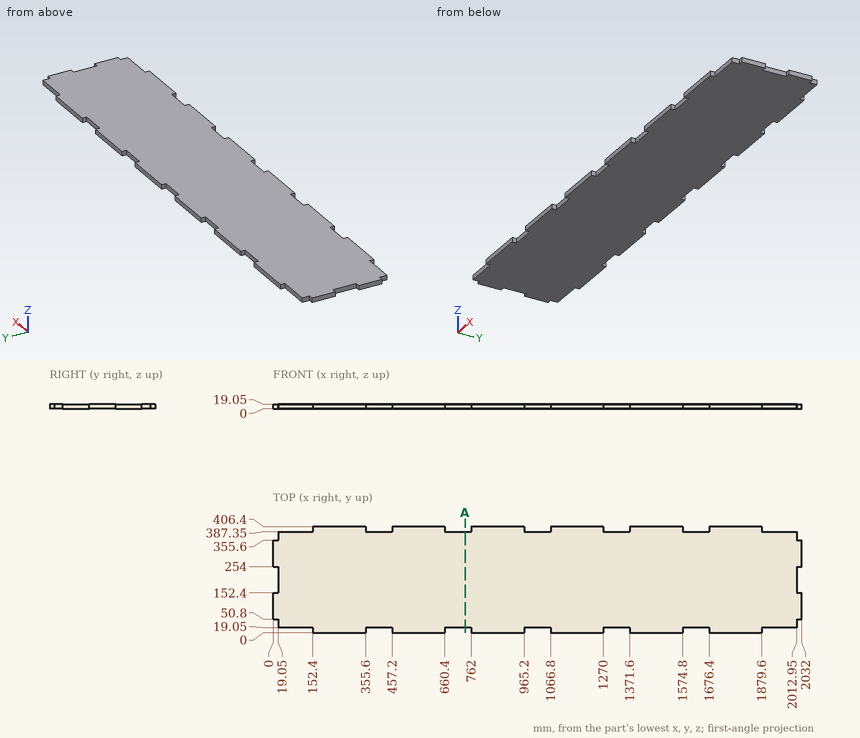
Geometry: see drawing. Coordinates: mm, zero at the bounding-box minimum. Coordinates: 2 decimals unless noted, no trailing zeros. Order: outer loops, then holes, each group sorted by start corner. A loop starts at its lowest first (then second) coordinate and runs counter-clockwise, first axis right, second up. Notation, with made-up numbers: (17.25, 68) - (25.25, 68) arc R10 ccw to (25.25, 77) - close; hole circle Ø5 at (23, 30.25). An arc over 180 degrees is marked (long way). Write each question's results on one line, items separated by ' | '.
1) Pin query (flat end, axial travel): pin 1 (5.5 mm diameter, centred on x = 2020, z = 6.5, fed in from -Y); pin 2 (3 mm diameter, centred on y = 44, z = 6, fed in from -X); pin 3 (10 mm diameter, centred on y = 304, z = 2.5, fed in from -X); pin 4 (8 mm diameter, centred on x = 1059, z = 16.5, fed in from -Y). Return the tip coordinate at first contact, or that it passes through.
Results list:
pin 1: y = 50.8 | pin 2: x = 19.05 | pin 3: x = 0 | pin 4: y = 19.05
2) Section A-A, the plane x = 738. Return loops of the section in (y, z).
Results list:
outline: (19.05, 0) - (387.35, 0) - (387.35, 19.05) - (19.05, 19.05) - close
3) Line query: line 1 (X direction, y = 18.5, z = 4.25); line 2 (Y direction, x = 1052, z = 14.75); line 3 (X direction, y = 42, z = 1.75). Output: solid intervals per line, ascending. Write a range as from..to.
Results list:
line 1: 152.4..355.6, 457.2..660.4, 762..965.2, 1066.8..1270, 1371.6..1574.8, 1676.4..1879.6 | line 2: 19.05..387.35 | line 3: 19.05..2012.95
